Can you work these out from the model? Positions are in its coordinate system, mm. A direction names the side the tool comes from. Round coordinates to 2 decimals unless told otherwise and drop trailing zeros. Loops run counter-clockwise (first coordinate to the right, second up) from the corner with the lowest first, then second, coordinate; pieces in that order, holes last. Notation, with made-up numbers: M -31,68 L -20,68 A19 cw -20,102 Z; hole C 36.5,49 d8. An arc over 180 degrees is marked long. Return JSON: item names as keys, results as strings.
Autodesk Fusion 360 part; units mm, degrees
sketch "Sketch1" plane through (0, 0, 0) normal (1, 0, 0) x (0, 1, 0)
  line L0 (0, 0) -> (0, 5)
  line L1 (0, 5) -> (12.6547, 39.7686)
  line L2 (0, 5) -> (37, 5) construction
  line L3 (12.6547, 39.7686) -> (32.6547, 39.7686)
  line L4 (32.6547, 39.7686) -> (32.6547, 0)
  line L5 (32.6547, 0) -> (0, 0)
  dimension "d1" = 70
  dimension "d2" = 37
  dimension "d3" = 20
extrude "Extrude1" add sketch "Sketch1" along normal mid plane 66
shell "Shell1" thickness 3 removed faces 1 at (11, 10.8849, 0)
chamfer "Chamfer1" distance 5 angle 45 1 edges at (0, 32.6547, 39.7686)
chamfer "Chamfer1" distance 0.5 angle 45 6 edges at (33, 22.6547, 39.7686) (-33, 22.6547, 39.7686) (0, 32.6547, 0) (33, 16.3274, 0) (0, 0, 0) (-33, 16.3274, 0)
fillet "Fillet1" radius 0.5 8 edges at (-33, 6.2364, 22.1343) (33, 6.2364, 22.1343) (-33, 32.6547, 17.6343) (33, 32.6547, 17.6343) (33, 30.4047, 37.0186) (-33, 30.4047, 37.0186) (-33, 0, 2.75) (33, 0, 2.75)
sketch "Sketch2" plane through (0, -1.607, 0.5849) normal (0, -0.9397, 0.342) x (1, 0, 0)
  line L0 (32.5, 4.6985) -> (32.5, 41.6985)
  line L1 (32.5, 41.6985) -> (-32.5, 41.6985)
  line L2 (-32.5, 41.6985) -> (-32.5, 4.6985)
  line L3 (-32.5, 4.6985) -> (32.5, 4.6985)
  line L4 (-32.5, 41.6985) -> (32.5, 4.6985) construction
  line L5 (32.5, 41.6985) -> (-32.5, 4.6985) construction
  line L6 (23, 40.2985) -> (-23, 40.2985)
  line L7 (-23, 40.2985) -> (-23, 6.0985)
  line L8 (-23, 6.0985) -> (23, 6.0985)
  line L9 (23, 6.0985) -> (23, 40.2985)
  line L10 (23, 40.2985) -> (-23, 6.0985) construction
  line L11 (-23, 40.2985) -> (23, 6.0985) construction
  point P0 (0, 23.1985)
  dimension "d13" = 46
  dimension "d14" = 34.2
extrude "Extrude2" cut sketch "Sketch2" against normal blind 6 contours L6 L7 L8 L9
Q1. Suppose I cut it at B-B, the plane x = 28.5. Please give me the cut outline in (y, z), plus the area to 3 significant figures.
Results:
{"outline": "M 0,0.5 L 0.5,0 L 3,0 L 3,4.47 L 14.76,36.77 L 29.65,36.77 L 29.65,0 L 32.15,0 L 32.65,0.5 L 32.65,34.77 L 27.65,39.77 L 12.65,39.77 L 0,5 Z", "area": "276 mm2"}
Q2. I'm going to push flat-ended pins straight in: pin 1 Ø10 at (x, z) = (12.5, 19.5) entering from -Y; pin 2 Ø2 at (x, z) = (-24.5, 6.5) entering from -Y; pin 3 Ø2 at (x, y) = (-20.5, 14.5) entering from -Z. Where does each tip first touch, or does it pass through?
Results:
{"pin 1": "stops at y = 29.65", "pin 2": "stops at y = 0.18", "pin 3": "stops at z = 37.24"}
Q3. Suppose I cut it at A-A, the plane x = 10.5. Please give me the cut outline in (y, z).
Results:
{"outline": "M 0,0.5 L 0.5,0 L 3,0 L 3,4.47 L 3.3,5.29 L 0.48,6.32 L 0,5 Z; M 12.18,38.45 L 16.8,36.77 L 29.65,36.77 L 29.65,0 L 32.15,0 L 32.65,0.5 L 32.65,34.77 L 27.65,39.77 L 12.65,39.77 Z"}
Q4. On a 3-axis mill with a long thin cutter (end or side, diameter ignored), from which of +Z, -Z, +X, -X, +Y, -Y can I reach the whole of each face in a straight line? I mean faces 1 (the flat face through (0.32, 14.46, 37.62)), 2 (the flat face through (2.08, 3.19, 4.99)), 3 (the flat face through (-0.3, 1.9, 5.8)), 4 (the flat face through (33, 20, 20)). Say none if no direction works.
Results:
{"face 1": "-Z, -Y", "face 2": "-Z", "face 3": "+Z", "face 4": "+Z, -Z, +X, +Y, -Y"}
Q5. Thinking about a two-plate mould opening in Y: for faces 5 (the flat face through (0, 20, 39.769)), 6 (the cylindrical face through (-32.86, 30.08, 37.13)), 7 (the cylindrical face through (-32.86, 6.56, 22.58)), 8 (the flat face through (0, 3, 2)), which applies, pulls with the +Y half, pulls with the -Y half, needs draft (parallel to the pull), parting line crosses it, or undercut?
Results:
{"face 5": "needs draft", "face 6": "pulls with the +Y half", "face 7": "pulls with the -Y half", "face 8": "undercut"}
Q6. Suppose I cut it at C-C, the plane y = 20. Please give me the cut outline in (x, z), plus the area to 3 significant figures.
Results:
{"outline": "M -33,0.5 L -32.5,0 L -30,0 L -30,36.77 L 30,36.77 L 30,0 L 32.5,0 L 33,0.5 L 33,39.27 L 32.5,39.77 L -32.5,39.77 L -33,39.27 Z", "area": "418 mm2"}
Q7. If I drill on line 1 along X through (y, z) = (15, 36); line 2 along X through (y, z) = (15, 37); line 3 along Y through (x, z) = (-12.5, 2), over which ranges is the centre line in solid material (lowest first)?
Results:
{"line 1": "x = -33 to -30, 30 to 33", "line 2": "x = -33 to -23, 23 to 33", "line 3": "y = 0 to 3, 29.65 to 32.65"}
